The model under review builds one solid part; all positions refer to its coordinate system, in mm. A direction names the side the tool comes from. Give positions to 0.01 mm unless a question says otherwise; leave off trailing zeros. Loops run counter-clockwise (first coordinate to the right, second up) from the corner with the lowest first, then second, coordinate; pieces in that order, holes last. Notation, with made-up numbers: M -24.75,-13 L 18.25,-13 A29 ccw 18.25,18 Z; hole C 69,-6.5 d6. An arc over 180 degrees is marked long. Put each result on its own line as item: value. Start each with the question number.
```python
from build123d import *

# Parameters (mm, degrees)
SKETCH2_W           = 34
SKETCH2_H           = 34
BOSS_EXTRUDE1_DEPTH = 5
SKETCH3_W           = 32
SKETCH3_H           = 32
CUT_EXTRUDE1_DEPTH  = 3
SKETCH4_R           = 1
BOSS_EXTRUDE2_DEPTH = 2
FILLET1_R           = 1


with BuildPart() as part:
    # Sketch2 → Boss-Extrude1 (new body)
    with BuildSketch(Plane(origin=(0, 0, 0), x_dir=(1, 0, 0), z_dir=(0, 1, 0))):
        Rectangle(SKETCH2_W, SKETCH2_H)
    extrude(amount=BOSS_EXTRUDE1_DEPTH)

    # Sketch3 → Cut-Extrude1 (cut)
    with BuildSketch(Plane.XZ):
        Rectangle(SKETCH3_W, SKETCH3_H)
    extrude(amount=-CUT_EXTRUDE1_DEPTH, mode=Mode.SUBTRACT)

    # Sketch4 → Boss-Extrude2 (add)
    with BuildSketch(Plane(origin=(0, 5, 0), x_dir=(1, 0, 0), z_dir=(0, 1, 0))):
        Circle(SKETCH4_R)
    extrude(amount=BOSS_EXTRUDE2_DEPTH)

    # Fillet1
    fillet1_edges = [part.edges().sort_by_distance(p)[0] for p in [
        (-1, 7, 0),
    ]]
    fillet(fillet1_edges, radius=FILLET1_R)


solid = part.part
```
Item 1: Consider section C-C, the plane x = -10.5. Write out the cut boundary in (y, z).
Item 2: Draft analysis for pull direction X (two halves, no side actions). For faces 1 (the cylindrical face through (-0.217, 5.493, 0.976)), 2 (the flat face through (17, 2, 0)), 3 (the flat face through (0, 3, 0)), state which applies: +X half, -X half, draft (parallel to the pull), parting line (faces both ways), or undercut.
Item 3: Consider section A-A, the plane z = 4. Write out the cut boundary in (x, y), plus the area to 3 significant figures.
Item 4: Consider section B-B, the plane y = 2.25. Write out the cut boundary in (x, z).
Item 5: Clearance check with flat-ended pins moving along their axes: pin 1 Ø17 at (x, z) = (-3.5, 3) entering from +Y; pin 2 Ø12 at (x, z) = (8.5, -5.5) entering from +Y; pin 3 Ø9.5 at (x, z) = (8, 7.5) entering from -Y. State where each tip first meets the part, or that it passes through.
Item 6: To check wall thickness, follow L1, parallel to Z at x = -2, y = 2; L2, parallel to Y at x = 9, z = 4.5. State the ranges of each line that lie inside material, in increasing order. Write a range as [from, to].
Item 7: Tool access review of faces 4 (the flat face through (16, 1, 0)), 5 (the flat face through (-1.3, 0, 16.3)): name each direction out of +Z, -Z, +X, -X, +Y, -Y from which nothing blocks a thin tool from reaching the whole face with its end or side.
Item 8: Consider section D-D, the plane y = 5.5. Write out the cut boundary in (x, z), plus the area to 3 significant figures.
Report:
1. outline: M 0,-17 L 5,-17 L 5,17 L 0,17 L 0,16 L 3,16 L 3,-16 L 0,-16 Z
2. face 1: parting line
2. face 2: +X half
2. face 3: undercut
3. outline: M -17,0 L -16,0 L -16,3 L 16,3 L 16,0 L 17,0 L 17,5 L -17,5 Z
3. area: 74.0 mm²
4. outline: M -17,-17 L 17,-17 L 17,17 L -17,17 Z; hole M -16,-16 L 16,-16 L 16,16 L -16,16 Z
5. pin 1: y = 7
5. pin 2: y = 5
5. pin 3: y = 3
6. L1: [-17, -16], [16, 17]
6. L2: [3, 5]
7. face 4: -Y
7. face 5: +Z, -Z, +X, -X, -Y
8. outline: C 0,0 d2
8. area: 3.14 mm²
